from build123d import *

# Parameters (mm, degrees)
SKETCH1_W           = 50
SKETCH1_H           = 30
BOSS_EXTRUDE1_DEPTH = 100
SKETCH1_3_W         = 50
SKETCH1_3_H         = 30
CUT_EXTRUDE1_DEPTH  = 30
SKETCH3_W           = 30
SKETCH3_H           = 40
CUT_EXTRUDE2_DEPTH  = 30


with BuildPart() as part:
    # Sketch1 → Boss-Extrude1 (new body)
    with BuildSketch(Plane.XY):
        with Locations((-50, 25)):
            Rectangle(SKETCH1_W, SKETCH1_H)
        Polygon((5, 40), (-25, 40), (-25, 10), (-75, 10), (-75, -40), (75, -40), (75, 0), align=None)
    extrude(amount=-BOSS_EXTRUDE1_DEPTH)

    # Sketch1_3 → Cut-Extrude1 (cut)
    with BuildSketch(Plane.XY):
        with Locations((-50, 25)):
            Rectangle(SKETCH1_3_W, SKETCH1_3_H)
    extrude(amount=-CUT_EXTRUDE1_DEPTH, mode=Mode.SUBTRACT)

    # Sketch3 → Cut-Extrude2 (cut)
    with BuildSketch(Plane(origin=(0, 40, 0), x_dir=(1, 0, 0), z_dir=(0, 1, 0))):
        with Locations((-60, 80)):
            Rectangle(SKETCH3_W, SKETCH3_H)
    extrude(amount=-CUT_EXTRUDE2_DEPTH, mode=Mode.SUBTRACT)


solid = part.part
CAD build for the part. Positions are in the model's coordinates, mm. A direction names the side the tool comes from. Round coordinates to 2 decimals unless told otherwise and drop trailing zeros. Order: outer loops, then holes, each group sorted by start corner. A loop starts at its lowest first (then second) coordinate and runs counter-clockwise, first axis right, second up. Notation, with made-up numbers: (70, -1) -> (125, -1) arc R8 ccw to (125, 12) -> close; hole circle Ø7 at (77, 18). An arc over 180 degrees is marked (long way). Write item = value, one per line. Start each with the question number.
(1) Cut at C-C, the plane x = -41.5. List the corners of the cut face in (y, z), then the cut area to 3 significant figures.
(2) Cut at D-D, the plane y = 30. List the corners of the cut face in (x, z), then the cut area to 3 significant figures.
(3) Cut at A-A, the plane y = 22. List the corners of the cut face in (x, z).
(4) Which spindle directions (+Z, -Z, +X, -X, +Y, -Y) get a long thin tool onto all of the face, cutting with end or side? Do faces 1 (the flat face through (-50, 25, -30)), 2 (the flat face through (-60, 10, -80)), 3 (the flat face through (-26, 40, -49)). Say none if no direction does.
(5) Cut at B-B, the plane z = -8. List the corners of the cut face in (x, y).
(6) Probe line 1 (Y direction, x = -54, z = -64); line 2 (Z direction, x = -39.5, y = 19.5); line 3 (X direction, y = 33, z = -58). List the from-to ranges inside material, lowest first. Write a range as [from, to].
(7) Pin check, flat tips, straight feed: P1, Ø24, axis at y = 32.5, z = -19.5, coming from the -X side; P2, Ø4, axis at y = 21, z = -58.5, coming from the +X side; P3, Ø15, axis at x = -38, y = 28, coming from the +Z side; P4, Ø9, axis at y = 24, z = -72, coming from the -X side. Stop position of each tip, or through.
Model answer:
q1.outline = (-40, -100) -> (40, -100) -> (40, -30) -> (10, -30) -> (10, 0) -> (-40, 0) -> close
q1.area = 7,100 mm2
q2.outline = (-75, -60) -> (-45, -60) -> (-45, -100) -> (22.5, -100) -> (22.5, 0) -> (-25, 0) -> (-25, -30) -> (-75, -30) -> close
q2.area = 7,050 mm2
q3.outline = (-75, -60) -> (-45, -60) -> (-45, -100) -> (36.5, -100) -> (36.5, 0) -> (-25, 0) -> (-25, -30) -> (-75, -30) -> close
q4.face_1 = +Z, -X, +Y
q4.face_2 = -Z, -X, +Y
q4.face_3 = +Z, -Z, +X, -X, +Y
q5.outline = (-75, -40) -> (75, -40) -> (75, 0) -> (5, 40) -> (-25, 40) -> (-25, 10) -> (-75, 10) -> close
q6.line_1 = [-40, 10]
q6.line_2 = [-100, -30]
q6.line_3 = [-75, 17.25]
q7.P1 = -75
q7.P2 = 41.75
q7.P3 = -30
q7.P4 = -45
